Geometry: final body of the model. Coordinates: model frame, mm. Face numbers are marked on the shaded views. A direction names the side the tool comes from. Coordinates: 2 decimals unless noted, no trailing zeros. Order: outer loops, then holes, each group sorted by start corner. A loop starts at its lowest first (then second) coordinate and runs counter-clockwise, first axis right, second up. Notation, with made-up numbers: (32.25, -32.75) -> (65.25, -32.75) arc R16 cw to (65.25, -12.75) -> close; hole circle Ø2 at (74, 64.25). An arc over 180 degrees is marked (long way). Use one line per item in the form item = value.
Autodesk Inventor part; units mm, degrees
ref_plane "작업 평면1" through (0, 10, 0) normal (0, 1, 0) x (1, 0, 0)
ref_plane "작업 평면2" through (0, 10, 0) normal (0, 1, 0) x (1, 0, 0)
ref_plane "작업 평면3" through (57.9435, 10, -25.2204) normal (0, 0, 1) x (1, 0, 0)
ref_plane "작업 평면1" through (0, 10, 0) normal (0, 1, 0) x (1, 0, 0)
sketch "스케치3" plane through (0, 10, 0) normal (0, 1, 0) x (1, 0, 0)
  line L0 (113.0685, 80.2704) -> (78.3685, 80.2704)
  line L1 (76.5185, 71.6407) -> (76.5185, 39.8907)
  line L2 (76.5185, 71.6407) -> (62.8185, 71.6407)
  line L3 (78.3685, 80.2704) -> (78.3685, 58.4704)
  line L4 (113.0685, 58.4704) -> (113.0685, 80.2704)
  line L5 (113.0685, 58.4704) -> (78.3685, 58.4704)
  line L6 (108.4435, 113.2704) -> (97.4435, 113.2704)
  line L7 (97.4435, 113.2704) -> (97.4435, 121.7204)
  line L8 (97.4435, 121.7204) -> (108.4435, 121.7204)
  line L9 (108.4435, 121.7204) -> (108.4435, 113.2704)
  line L10 (113.0685, 52.4704) -> (78.3685, 52.4704)
  line L11 (113.0685, 30.6704) -> (113.0685, 52.4704)
  line L12 (62.8185, 39.8907) -> (76.5185, 39.8907)
  line L13 (62.8185, 71.6407) -> (62.8185, 39.8907)
  line L14 (78.3685, 52.4704) -> (78.3685, 30.9204)
  line L15 (113.0685, 30.6704) -> (78.3685, 30.9204)
  line L16 (117.9435, 121.7204) -> (57.9435, 121.7204)
  line L17 (57.9435, 121.7204) -> (57.9435, 11.7204)
  line L18 (117.9435, 11.7204) -> (117.9435, 121.7204)
  line L19 (57.9435, 11.7204) -> (117.9435, 11.7204)
  circle A0 centre (87.9435, 108.2204) radius 2.25
  circle A1 centre (87.9435, 25.2204) radius 2.25
  line L20 (113.0685, 99.0204) -> (108.0685, 99.0204)
  line L21 (108.0685, 90.0204) -> (113.0685, 90.0204)
  line L22 (113.0685, 99.0204) -> (113.0685, 90.0204)
  line L23 (108.0685, 99.0204) -> (108.0685, 90.0204)
  line L24 (71.9185, 39.8907) -> (67.4185, 39.8907)
  line L25 (113.0685, 39.3204) -> (108.0685, 39.3204)
  line L26 (108.0685, 43.8204) -> (113.0685, 43.8204)
  line L27 (71.9185, 44.8907) -> (71.9185, 39.8907)
  line L28 (108.0685, 43.8204) -> (108.0685, 39.3204)
  line L29 (113.0685, 43.8204) -> (113.0685, 39.3204)
  line L30 (71.9185, 44.8907) -> (67.4185, 44.8907)
  line L31 (67.4185, 44.8907) -> (67.4185, 39.8907)
  line L32 (113.0685, 71.6204) -> (113.0685, 67.1204)
  line L33 (113.0685, 86.2704) -> (89.4185, 86.2704)
  line L34 (89.4185, 86.2704) -> (89.4185, 102.7704)
  line L35 (89.4185, 102.7704) -> (113.0685, 102.7704)
  line L36 (113.0685, 102.7704) -> (113.0685, 86.2704)
  line L37 (108.0685, 67.1204) -> (113.0685, 67.1204)
  line L38 (113.0685, 67.1204) -> (113.0685, 71.6204)
  line L39 (113.0685, 71.6204) -> (108.0685, 71.6204)
  line L40 (108.0685, 71.6204) -> (108.0685, 67.1204)
  line L41 (113.0685, 30.6704) -> (108.0685, 30.6704)
  line L42 (108.0685, 30.6704) -> (108.0685, 52.4704)
  line L43 (108.0685, 52.4704) -> (113.0685, 52.4704)
  line L44 (113.0685, 52.4704) -> (113.0685, 30.6704)
  line L45 (113.0685, 58.4704) -> (108.0685, 58.4704)
  line L46 (108.0685, 58.4704) -> (108.0685, 80.2704)
  line L47 (108.0685, 80.2704) -> (113.0685, 80.2704)
  line L48 (113.0685, 80.2704) -> (113.0685, 58.4704)
  line L49 (113.0685, 86.2704) -> (108.0685, 86.2704)
  line L50 (108.0685, 86.2704) -> (108.0685, 102.7704)
  line L51 (108.0685, 102.7704) -> (113.0685, 102.7704)
  line L52 (113.0685, 102.7704) -> (113.0685, 86.2704)
  line L53 (76.5185, 39.8907) -> (62.8185, 39.8907)
  line L54 (62.8185, 39.8907) -> (62.8185, 44.8907)
  line L55 (62.8185, 44.8907) -> (76.5185, 44.8907)
  line L56 (76.5185, 44.8907) -> (76.5185, 39.8907)
  point P0 (0, 0)
  dimension "d8" = 9.5
extrude "돌출2" add sketch "스케치3" against normal blind 10 contours L4 L39 L46 L0 | L46 L40 L5 L3 L0 | L4 L37 L40 L39 | L4 L5 L46 L37 | L1 L55 L30 L13 L2 | L1 L12 L27 L55 | L27 L12 L31 L30 | L55 L31 L12 L13 | L9 L16 L18 L19 L17 L7 L6 | L6 L7 L8 L9 | L11 L26 L42 L10 | L42 L28 L15 L14 L10 | L11 L25 L28 L26 | L11 L15 L42 L25 | L41 L42 L15 | A0 | A1 | L22 L21 L23 L20 | L20 L50 L35 L36 | L23 L50 L33 L34 L35 | L36 L33 L50 L21
sketch "스케치4" plane through (0, 10, 0) normal (0, 1, 0) x (1, 0, 0)
  point P0 (0, 0)
extrude "돌출3" cut sketch "스케치3" against normal blind 1.7 contours L4 L39 L46 L0 | L46 L40 L5 L3 L0 | L4 L5 L46 L37 | L1 L55 L30 L13 L2 | L1 L12 L27 L55 | L55 L31 L12 L13 | L11 L26 L42 L10 | L42 L28 L15 L14 L10 | L11 L15 L42 L25 | L20 L50 L35 L36 | L23 L50 L33 L34 L35 | L36 L33 L50 L21
extrude "돌출4" cut sketch "스케치3" against normal through all contours L4 L37 L40 L39 | L27 L12 L31 L30 | L11 L25 L28 L26 | A0 | A1 | L22 L21 L23 L20
sketch "스케치5" plane through (117.9435, 10, -121.7204) normal (0, 0, -1) x (-1, 0, 0)
  point P0 (117.9435, -10)
extrude "돌출5" cut sketch "스케치3" against normal through all contours L6 L7 L8 L9
sketch "스케치6" plane through (0, 0, 0) normal (0, -1, 0) x (1, 0, 0)
  line L0 (57.9435, -121.7204) -> (97.4435, -121.7204)
  line L1 (97.4435, -121.7204) -> (57.9435, -121.7204)
  line L2 (113.0685, -71.6204) -> (108.0685, -71.6204)
  line L3 (113.0685, -80.2704) -> (113.0685, -71.6204)
  line L4 (78.3685, -80.2704) -> (113.0685, -80.2704)
  line L5 (78.3685, -58.4704) -> (78.3685, -80.2704)
  line L6 (113.0685, -58.4704) -> (78.3685, -58.4704)
  line L7 (113.0685, -67.1204) -> (113.0685, -58.4704)
  line L8 (108.0685, -67.1204) -> (113.0685, -67.1204)
  line L9 (108.0685, -71.6204) -> (108.0685, -67.1204)
  line L10 (117.9435, -121.7204) -> (108.4435, -121.7204)
  line L11 (111.4435, -108.7204) -> (94.443, -108.7204)
  line L12 (111.4435, -108.7204) -> (111.4435, -113.2704)
  line L13 (94.443, -108.7204) -> (94.443, -113.2704)
  line L14 (111.4435, -113.2704) -> (94.443, -113.2704)
  point P0 (0, 0)
sketch "스케치7" plane through (0, 0, 0) normal (0, -1, 0) x (1, 0, 0)
  point P0 (0, 0)
sketch "스케치8" plane through (0, 0, 0) normal (0, -1, 0) x (1, 0, 0)
  point P0 (0, 0)
extrude "돌출6" cut sketch "스케치6" against normal blind 4 contours L12 L14 L13 L11
extrude "돌출7" add sketch "스케치3" against normal blind 6 contours L6 L7 L8 L9
sketch "스케치9" plane through (0, 0, 0) normal (0, -1, 0) x (1, 0, 0)
  line L0 (111.4435, -108.7204) -> (111.4435, -113.2704)
  line L1 (111.4435, -108.7204) -> (111.4435, -101.7204)
  line L2 (111.4435, -101.7204) -> (94.443, -101.7204)
  line L3 (94.443, -113.2704) -> (94.443, -108.7204)
  line L4 (94.443, -101.7204) -> (94.443, -108.7204)
  line L5 (94.443, -108.7204) -> (111.4435, -108.7204)
  line L6 (111.4435, -108.7204) -> (94.443, -108.7204)
  point P0 (0, 0)
  dimension "d25" = 7
extrude "돌출8" cut sketch "스케치9" against normal blind 4
sketch "스케치10" plane through (0, 10, 0) normal (0, 1, 0) x (1, 0, 0)
  circle A0 centre (87.9435, 25.2204) radius 2.25
  circle A1 centre (87.9435, 25.2204) radius 3.85
  circle A2 centre (87.9435, 108.2204) radius 2.25
  circle A3 centre (87.9435, 108.2204) radius 3.85
  point P0 (0, 0)
  dimension "d28" = 7.7
  dimension "d29" = 7.7
ref_plane "작업 평면2" through (0, 10, 0) normal (0, 1, 0) x (1, 0, 0)
sketch "스케치12" plane through (0, 10, 0) normal (0, 1, 0) x (1, 0, 0)
  point P0 (0, 0)
ref_plane "작업 평면3" through (57.9435, 10, -25.2204) normal (0, 0, 1) x (1, 0, 0)
sketch "스케치13" plane through (57.9435, 10, -25.2204) normal (0, 0, 1) x (1, 0, 0)
  line L0 (30, 0) -> (30, -4)
  line L1 (30, 0) -> (33.65, 0)
  line L2 (27.75, 0) -> (32.25, 0)
  line L3 (33.65, 0) -> (30, -4)
  point P0 (-57.9435, -10)
  dimension "d35" = 4
  dimension "d36" = 3.65
sketch "스케치14" plane through (57.9435, 10, -25.2204) normal (0, 0, 1) x (1, 0, 0)
  point P0 (-57.9435, -10)
revolve "회전2" cut sketch "스케치13" angle 360 about axis through (87.9435, 10, -25.2204) along (0, -1, 0)
ref_plane "작업 평면4" through (57.9435, 10, -66.7204) normal (0, 0, 1) x (1, 0, 0)
mirror "미러1" about plane through (57.9435, 10, -66.7204) normal (0, 0, 1) of "회전2"
sketch "스케치15" plane through (0, 0, 0) normal (0, -1, 0) x (1, 0, 0)
  line L0 (108.6612, -121.7204) -> (97.1612, -121.7204)
  line L1 (97.1612, -121.7204) -> (97.1612, -113.2704)
  line L2 (108.6612, -121.7204) -> (108.6612, -113.2704)
  line L3 (97.1612, -113.2704) -> (108.6612, -113.2704)
  line L4 (97.4435, -113.2704) -> (94.443, -113.2704)
  point P0 (0, 0)
extrude "돌출9" cut sketch "스케치15" against normal blind 4
extrude "돌출10" cut sketch "스케치3" against normal through all contours L4 L39 L46 L0 | L4 L5 L46 L37 | L1 L12 L27 L55 | L55 L31 L12 L13 | L11 L26 L42 L10 | L11 L15 L42 L25 | L41 L42 L15 | L20 L50 L35 L36 | L36 L33 L50 L21
equation "\"TransitionRadius\" = BendRadius"
properties part number "123"
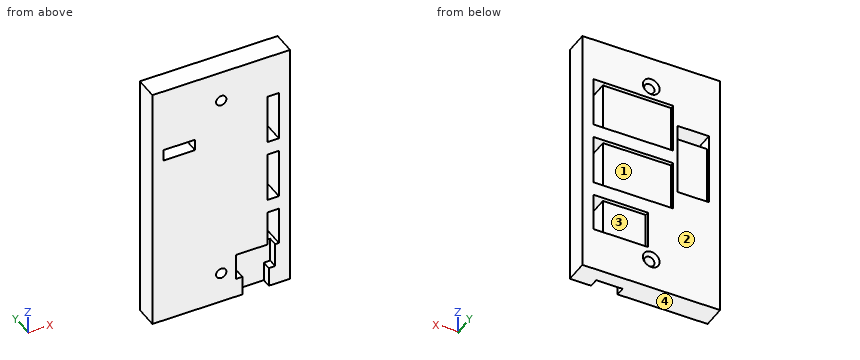
1) Contact query for flat-ended pins moving along their axis: P1, Ø11, axis at x = 73, z = -61.5, coming from the +Y side; P2, Ø17.5, axis at x = 97.5, z = -69.5, coming from the +Y side. Output: stop coordinate, or through.
Results found:
P1 = 10
P2 = 8.3
2) Access query for the marked faces 1 and 2. Directions: +Z, -Z, +X, -X, +Y, -Y. A direction counts if a zero-diameter tool reaches every point of the face in a straight line with its end or side. Return the directions, or none.
Results found:
face_1 = +Y
face_2 = +Z, -Z, +X, -X, +Y
3) Section D-D, the plane z = -68. Output: boundary loops of the cut face in (x, y), and give its area (3 significant figures).
Results found:
outline = (57.94, 0) -> (108.07, 0) -> (108.07, 8.3) -> (78.37, 8.3) -> (78.37, 10) -> (76.52, 10) -> (76.52, 8.3) -> (62.82, 8.3) -> (62.82, 10) -> (57.94, 10) -> close; (113.07, 0) -> (117.94, 0) -> (117.94, 10) -> (113.07, 10) -> close
area = 476 mm2
4) Material intervals for probe 1 along X at (y, z) = (7, -43); probe 2 along X at (y, z) = (9, -96.5); probe 3 along Z at (x, y) = (65.5, 1), sorted ascending. Write a range as from..to.
Results found:
probe_1 = 57.94..62.82, 76.52..108.07, 113.07..117.94
probe_2 = 57.94..89.42, 113.07..117.94
probe_3 = -121.72..-44.89, -39.89..-11.72
5) Section B-B, the plane z = -96. Output: boundary loops of the cut face in (x, y), and give its area (3 significant figures).
Results found:
outline = (57.94, 0) -> (108.07, 0) -> (108.07, 8.3) -> (89.42, 8.3) -> (89.42, 10) -> (57.94, 10) -> close; (113.07, 0) -> (117.94, 0) -> (117.94, 10) -> (113.07, 10) -> close
area = 518 mm2
6) Pull-direction query (X, two-part tool) for the marked faces 3 and 4; classes: released by +X, released by -X, zero draft, split by the parting line, or undercut.
Results found:
face_3 = undercut
face_4 = zero draft
7) Section A-A, the plane x = 73.5. Output: boundary loops of the cut face in (y, z), and give its area (3 significant figures).
Results found:
outline = (0, -121.72) -> (10, -121.72) -> (10, -71.64) -> (8.3, -71.64) -> (8.3, -44.89) -> (0, -44.89) -> close; (0, -39.89) -> (10, -39.89) -> (10, -11.72) -> (0, -11.72) -> close
area = 1,000 mm2
8) Section C-C, the plane y = 2. Give the number of separate pieces and of enclosed holes in the cut face, and give its area (3 significant figures).
Results found:
separate_pieces = 1
enclosed_holes = 5
area = 5,910 mm2
